```python
from build123d import *

# Parameters (mm, degrees)
F0_W     = 35
F0_H     = 25
F1_DEPTH = 4
F2_W     = 26
F2_H     = 5.5
F3_DEPTH = 3.2
F4_W     = 26
F4_H     = 5.5
F5_DEPTH = 3.8


with BuildPart() as f1:
    # F0 (on Top) → F1 (new body)
    with BuildSketch(Plane.XY):
        with Locations((-17.5, 2.854638)):
            Rectangle(F0_W, F0_H)
    extrude(amount=F1_DEPTH)

    # F2 (on face) → F3 (join)
    with BuildSketch(Plane.XY.offset(4)):
        with Locations((-22, 8.104638)):
            Rectangle(F2_W, F2_H)
    extrude(amount=F3_DEPTH)

    # F4 (on face) → F5 (join)
    with BuildSketch(Plane.XY.offset(7.2)):
        with BuildLine():
            Line((-35, 5.354638), (-35, 3.204638))
            Line((-35, 3.204638), (-8.4, 3.204638))
            ThreePointArc((-8.4, 3.204638), (-4.935177, 4.639814), (-3.5, 8.104638))
            ThreePointArc((-3.5, 8.104638), (-4.935177, 11.569461), (-8.4, 13.004638))
            Line((-8.4, 13.004638), (-35, 13.004638))
            Line((-35, 13.004638), (-35, 10.854638))
            Line((-35, 10.854638), (-9, 10.854638))
            Line((-9, 10.854638), (-9, 5.354638))
            Line((-9, 5.354638), (-35, 5.354638))
        make_face()
        with Locations((-22, 8.104638)):
            Rectangle(F4_W, F4_H)
    extrude(amount=F5_DEPTH)


solid = f1.part
```
Geometry: final body of the model. Coordinates: model frame, mm. A direction names the side the tool comes from. Round coordinates to 2 decimals unless told otherwise and drop trailing zeros. Order: outer loops, then holes, each group sorted by start corner. A loop starts at its lowest first (then second) coordinate and runs counter-clockwise, first axis right, second up. Notation, with made-up numbers: (28.25, 49) -> (64.25, 49) arc R31 ccw to (64.25, 85) -> close; hole circle Ø2 at (-17, 38). An arc over 180 degrees is marked (long way). Use one line per item in the form item = value. Start each with the question number.
1. Pin query (flat end, axial travel): pin 1 Ø5 at (x, y) = (-4, -0.5) entering from +Z; pin 2 Ø3 at (x, y) = (-25.5, -4.5) entering from -Z; pin 3 Ø6 at (y, z) = (2.5, 10) entering from +X; pin 4 Ø4 at (x, z) = (-26, 9.5) entering from +Y. Return the tip coordinate at first contact, or that it passes through.
2. Cut plane A-A (x = -12). Return the cut outline in (y, z), then the cut area to 3 significant figures.
3. Cut plane C-C (y = -1.75). Return the cut outline in (x, z), then the cut area to 3 significant figures.
4. Draft query along Z for faces 4 (the face through (-35, 6, 4)), 5 (the face through (-9, 8, 6)), 6 (the face through (-18, 3, 0)). Return one class per face: pulls with the +Z half, pulls with the -Z half, needs draft (parallel to the pull), parting line crosses it, or undercut.
5. Cut plane D-D (y = 9.5). Return the cut outline in (x, z).
6. Cut plane B-B (z = 10). Return the cut outline in (x, y), then the cut area to 3 significant figures.
7. Line query: probe 1 along Z at (x, y) = (-5.5, 5.25); probe 2 along Y at (x, z) = (-29.5, 8.25); probe 3 along Y at (x, z) = (-27.5, 6). Output: solid intervals per line, ascending.
8. Reachability of faces 1 (the face through (-22, 13.005, 9)), 2 (the face through (-22, 3.205, 9)), 3 (the face through (-22, 10.855, 6)) from +Z, -Z, +X, -X, +Y, -Y: full face, straight path, thin tool, end or side. Return the list, or none.
Solution:
q1.pin_1 = 4
q1.pin_2 = 0
q1.pin_3 = -4.25
q1.pin_4 = 13
q2.outline = (-9.65, 0) -> (15.35, 0) -> (15.35, 4) -> (10.85, 4) -> (10.85, 7.2) -> (13, 7.2) -> (13, 11) -> (3.2, 11) -> (3.2, 7.2) -> (5.35, 7.2) -> (5.35, 4) -> (-9.65, 4) -> close
q2.area = 155 mm^2
q3.outline = (-35, 0) -> (0, 0) -> (0, 4) -> (-35, 4) -> close
q3.area = 140 mm^2
q4.face_4 = needs draft
q4.face_5 = undercut
q4.face_6 = pulls with the -Z half
q5.outline = (-35, 0) -> (0, 0) -> (0, 4) -> (-9, 4) -> (-9, 7.2) -> (-3.7, 7.2) -> (-3.7, 11) -> (-35, 11) -> close
q6.outline = (-35, 3.2) -> (-8.4, 3.2) arc R4.9 ccw to (-3.5, 8.1) arc R4.9 ccw to (-8.4, 13) -> (-35, 13) -> close
q6.area = 298 mm^2
q7.probe_1 = 0 to 4, 7.2 to 11
q7.probe_2 = 3.2 to 13
q7.probe_3 = 5.35 to 10.85
q8.face_1 = +Z, +X, -X, +Y
q8.face_2 = +Z, +X, -X, -Y
q8.face_3 = +X, -X, +Y
